For this review, take the finished solid that the model builds, in its own axes (mm). A direction names the side the tool comes from. Coordinates: 2 decimals unless noted, no trailing zeros. Order: outer loops, then holes, each group sorted by start corner. A loop starts at its lowest first (then second) coordinate and runs counter-clockwise, first axis right, second up. Notation, with made-up numbers: (72.5, -28.5) -> (85.5, -28.5) arc R17 ccw to (85.5, -17.5) -> close; hole circle Ø11 at (13, 32). An arc over 180 degrees is marked (long way). Answer as a JSON object with one key per item and string values. Group by question number.
1) Add section D-D, the plane x = -28. Write out the cut boundary in (y, z), then the cut area to 3 significant figures.
2) Add section B-B, the plane y = 0. Write out the cut boundary in (x, z) (1 decimal), then the cut area to 3 significant figures.
3) Draft analysis for pull direction Z (two halves, no side actions). For faces 1 (the flat face through (-6, 25.4, 77)), 2 (the flat face through (-7, -4, 82)), 3 (the flat face through (-64, -1, 12.7)), state which applies: +Z half, -Z half, draft (parallel to the pull), parting line (faces both ways), or undercut.
4) Machinability: for faces 4 (the cylindrical face through (-11.917, -0.279, 139.697)), 5 (the flat face through (-12.7, 50, 6)), 6 (the flat face through (-12.7, -51, 6)), which of the approach directions +Z, -Z, +X, -X, +Y, -Y give a long, thin tool a straight path to every point of the face, cutting with its end or side? Answer none if there is none.
5) For pin 1 (15 mm diameter, centred on y = -11, z = 70, fed in from -X); pin 2 (6.5 mm diameter, centred on y = -3, z = 107, fed in from +X) (3 decimals); pin 3 (6.5 mm diameter, centred on y = 53.5, z = 6, fed in from +X), all flat-tipped, find the tip position at first contact; note any pin that passes through.
6) Wall thickness on L1, parallel to X at y = 5, z = 45 (1 decimal); L2, parallel to Z at x = -47, y = -64; L3, parallel to X at y = 31.5, z = 12: over which ranges is each line inside the solid? List them lowest first.
from build123d import *

# Parameters (mm, degrees)
F1_DEPTH = 25.4
F0_W     = 101.6
F0_H     = 12.7
F2_DEPTH = 76.2
F3_W     = 3.175
F3_H     = 12.7
F4_DEPTH = 152.4
F6_DEPTH = 12.701
F7_DEPTH = 1.5875


with BuildPart() as f1:
    # F0 (on Front) → F1 (new body, symmetric)
    with BuildSketch(Plane.XZ):
        Polygon((-12.7, 0), (0, 0), (0, 152.4), (-12.7, 152.4), (-12.7, 12.7), align=None)
    extrude(amount=F1_DEPTH, both=True)

    # F0 (on Front) → F2 (join, symmetric)
    with BuildSketch(Plane.XZ):
        with Locations((-63.5, 6.35)):
            Rectangle(F0_W, F0_H)
    extrude(amount=F2_DEPTH, both=True)

    # F3 (on face) → F4 (cut, through all)
    with BuildSketch(Plane(origin=(0, 0, 0), x_dir=(1, 0, 0), z_dir=(0, 0, -1))):
        with Locations((-1.5875, 0)):
            Rectangle(F3_W, F3_H)
    extrude(amount=-F4_DEPTH, mode=Mode.SUBTRACT)

    # F5 (on face) → F6 (cut, through all)
    with BuildSketch(Plane(origin=(-12.7, 0, 0), x_dir=(0, -1, 0), z_dir=(-1, 0, 0))):
        with BuildLine():
            ThreePointArc((-4, 38.1), (0, 34.1), (4, 38.1))
            Line((4, 38.1), (4, 127))
            ThreePointArc((4, 127), (0, 131), (-4, 127))
            Line((-4, 127), (-4, 38.1))
        make_face()
    extrude(amount=-F6_DEPTH, mode=Mode.SUBTRACT)

    # F5 (on face) → F7 (cut)
    with BuildSketch(Plane(origin=(-12.7, 0, 0), x_dir=(0, -1, 0), z_dir=(-1, 0, 0))):
        with BuildLine():
            ThreePointArc((-12.7, 38.1), (0, 25.4), (12.7, 38.1))
            Line((12.7, 38.1), (12.7, 127))
            ThreePointArc((12.7, 127), (0, 139.7), (-12.7, 127))
            Line((-12.7, 127), (-12.7, 38.1))
        make_face()
        with BuildLine():
            Line((4, 127), (4, 38.1))
            ThreePointArc((4, 38.1), (0, 34.1), (-4, 38.1))
            Line((-4, 38.1), (-4, 127))
            ThreePointArc((-4, 127), (0, 131), (4, 127))
        make_face(mode=Mode.SUBTRACT)
    extrude(amount=-F7_DEPTH, mode=Mode.SUBTRACT)


solid = f1.part
Output values:
{
 "1": {"outline": "(-76.2, 0) -> (76.2, 0) -> (76.2, 12.7) -> (-76.2, 12.7) -> close", "area": "1,940 mm²"},
 "2": {"outline": "(-114.3, 0) -> (-3.2, 0) -> (-3.2, 34.1) -> (-11.1, 34.1) -> (-11.1, 25.4) -> (-12.7, 25.4) -> (-12.7, 12.7) -> (-114.3, 12.7) -> close; (-12.7, 139.7) -> (-11.1, 139.7) -> (-11.1, 131) -> (-3.2, 131) -> (-3.2, 152.4) -> (-12.7, 152.4) -> close", "area": "1,790 mm²"},
 "3": {"face 1": "draft", "face 2": "undercut", "face 3": "+Z half"},
 "4": {"face 4": "-X", "face 5": "+Z, -Z, +X, +Y", "face 6": "+Z, -Z, +X, -Y"},
 "5": {"pin 1": "stops at x = -12.7", "pin 2": "stops at x = -3.175", "pin 3": "stops at x = -12.7"},
 "6": {"L1": "x = -11.1 to -3.2", "L2": "z = 0 to 12.7", "L3": "x = -114.3 to -12.7"}
}
